from build123d import *

# Parameters (mm, degrees)
SKETCH1_W           = 342.543491
SKETCH1_H           = 161.067786
BOSS_EXTRUDE1_DEPTH = 54
SKETCH3_R           = 9
CUT_EXTRUDE1_DEPTH  = 340.02
SKETCH4_R           = 15
SKETCH4_R_2         = 12.5
BOSS_EXTRUDE2_DEPTH = 3


with BuildPart() as part:
    # Sketch1 → Boss-Extrude1 (new body)
    with BuildSketch(Plane(origin=(0, 0, 0), x_dir=(1, 0, 0), z_dir=(0, 1, 0))):
        Rectangle(SKETCH1_W, SKETCH1_H)
    extrude(amount=BOSS_EXTRUDE1_DEPTH)

    # Sketch3 → Cut-Extrude1 (cut)
    with BuildSketch(Plane(origin=(0, 0, -80.533893), x_dir=(-1, 0, 0), z_dir=(0, 0, -1))):
        with Locations((-105.2849429, 27)):
            Circle(SKETCH3_R)
        with Locations((105.2849429, 27)):
            Circle(SKETCH3_R)
    extrude(amount=-CUT_EXTRUDE1_DEPTH, mode=Mode.SUBTRACT)

    # Sketch4 → Boss-Extrude2 (add)
    with BuildSketch(Plane(origin=(0, 54, 0), x_dir=(1, 0, 0), z_dir=(0, 1, 0))):
        with Locations((-81.2717455, 0)):
            Circle(SKETCH4_R)
        with Locations((-81.2717455, 0)):
            Circle(SKETCH4_R_2, mode=Mode.SUBTRACT)
    extrude(amount=BOSS_EXTRUDE2_DEPTH)


solid = part.part
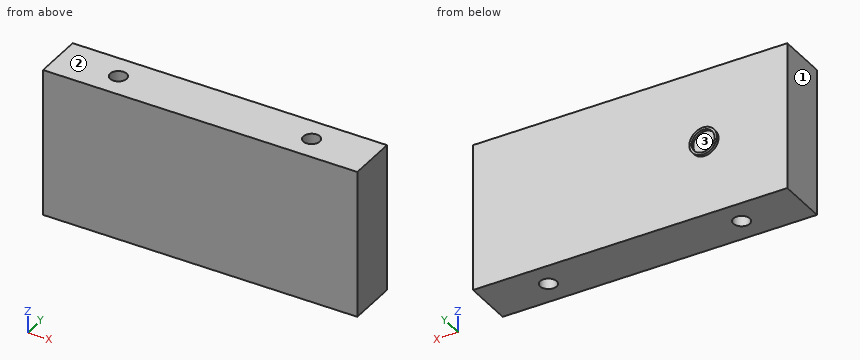
Can you work these out from the model? Positions are in its coordinate system, mm. Face numbers are marked on the shaded views. Give positions to 0.01 mm unless a question says otherwise; leave off trailing zeros. Loops run counter-clockwise (first coordinate to the right, second up) from the corner with the lowest first, then second, coordinate; pieces in that order, holes last. Notation, with made-up numbers: M -15,-35 L 11,-35 A19 cw 11,2 Z; hole C 18.25,62.5 d8. An arc over 180 degrees is marked long. One line per item, written item: value.
1) Imagine slicing it at C-C on x = -147.5. Write out the boundary of the cut face in (y, z), and give its area (3 significant figures).
Geometry check:
outline: M 0,-80.53 L 54,-80.53 L 54,80.53 L 0,80.53 Z
area: 8,700 mm²
2) Imagine slicing it at B-B on y = 27. Write out the boundary of the cut face in (x, z), and give its area (3 significant figures).
Geometry check:
outline: M -171.27,-80.53 L -114.28,-80.53 L -114.28,80.53 L -171.27,80.53 Z; M -96.28,-80.53 L 96.28,-80.53 L 96.28,80.53 L -96.28,80.53 Z; M 114.28,-80.53 L 171.27,-80.53 L 171.27,80.53 L 114.28,80.53 Z
area: 49,400 mm²
3) Imagine slicing it at A-A on z = 0. Write out the boundary of the cut face in (x, y), and give its area (3 significant figures).
Geometry check:
outline: M -171.27,0 L 171.27,0 L 171.27,54 L -66.27,54 L -66.27,57 L -68.77,57 L -68.77,54 L -93.77,54 L -93.77,57 L -96.27,57 L -96.27,54 L -171.27,54 Z; hole C -105.28,27 d18; hole C 105.28,27 d18
area: 18,000 mm²
4) I'm going to push flat-ended pins straight in: pin 1 (7.5 mm diameter, centred on x = -76, z = 2, fed in from +Y); pin 2 (14.5 mm diameter, centred on x = 105.28, y = 27, fed in from +Z). Where does each tip first touch, or does it pass through?
Geometry check:
pin 1: stops at y = 54
pin 2: passes through
5) Thinking about a two-plate mould opening in X: for the marked faces 1, 2 and 3, which applies, +X half, -X half, draft (parallel to the pull), parting line (faces both ways), or undercut?
Geometry check:
face 1: -X half
face 2: draft
face 3: undercut
6) Imagine slicing it at D-D on z = -38. Write out the boundary of the cut face in (x, y).
Geometry check:
outline: M -171.27,0 L 171.27,0 L 171.27,54 L -171.27,54 Z; hole C -105.28,27 d18; hole C 105.28,27 d18
7) Please list where these lines run through material, in increasing order: line 1 (X direction, y = 28, z = 29.5); line 2 (X direction, y = 54.9, z = 0); line 3 (X direction, y = 24, z = 26.5).
Geometry check:
line 1: x = -171.27 to -114.23, -96.34 to 96.34, 114.23 to 171.27
line 2: x = -96.27 to -93.77, -68.77 to -66.27
line 3: x = -171.27 to -113.77, -96.8 to 96.8, 113.77 to 171.27
